Check sheet for the modelled part. Datum: model origin and axes. Units: mm. Face numbers are marked on the shaded views. A direction names the side the tool comes from. Round coordinates to 2 decimals unless told otherwise and drop trailing zeros. Loops run counter-clockwise (first coordinate to the right, second up) from the corner with the lowest first, then second, coordinate; pieces in that order, holes last. Notation, with made-up numbers: (-22, 12) - (-8, 12) arc R26 cw to (-8, 32) - close; hole circle Ø11 at (6, -30.75). An arc over 180 degrees is marked (long way). Answer in a Markdown table with one row per item. Add a question column.
(1) Cross-section at A-A on x = 2. Enter the section's corners in (y, z) (3 decimals), then the cut area to 3 significant figures.
(2) Gauge pin test, flat ends, axial feed: pin 1 (8.5 mm diameter, centred on x = 24, z = 22, fed in from -Y) (3 decimals); pin 2 (5 mm diameter, centred on x = -120, y = -122.125, fed in from -Z); pin 3 (6 mm diameter, centred on x = 24, z = 110, fed in from +Y) (3 decimals); pin 4 (4 mm diameter, centred on x = -24, z = 22, fed in from -Y) (3 decimals). Record the tip position at first contact, or that the pin passes through.
(3) Cross-section at B-B on x = -120. Enter the section's corners in (y, z) (3 decimals).
(4) Cross-section at D-D on z = 41.5. Enter the section's corners in (x, y) (3 decimals).
(5) Access from +Z, -Z, +X, -X, +Y, -Y to the whole of each face (thin tool, end or side, straight path). Record for the marked faces 4, 5, 6, 7 and 8.
(6) Cross-section at C-C on y = 74. Enter the section's corners in (x, z).
(7) Mould release check, pull along X, two halves, no side actions. Record for the marked faces 1, 2 and 3: +X half, -X half, draft (parallel to the pull), parting line (faces both ways), or undercut.
(8) Thickness scan on line 1 along Y through (x, z) = (120, 123) (3 decimals); line 2 along X through (y, z) = (-95, 89.5); line 3 along Z through (x, y) = (-98, 122). Record the ranges inside material, lowest first.
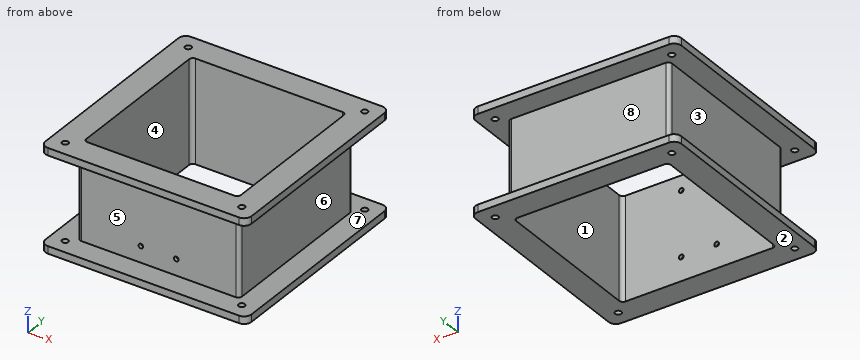
from build123d import *

# Parameters (mm, degrees)
SKETCH_4_W                  = 220
SKETCH_4_H                  = 224.25
SKETCH_4_W_2                = 210
SKETCH_4_H_2                = 214.25
EXTRUDE_7_DEPTH             = 120
SKETCH_7_W                  = 280
SKETCH_7_H                  = 284.25
SKETCH_7_W_2                = 210
SKETCH_7_H_2                = 214.25
EXTRUDE_8_DEPTH             = 10
SKETCH_8_W                  = 280
SKETCH_8_H                  = 284.25
SKETCH_8_W_2                = 210
SKETCH_8_H_2                = 214.25
EXTRUDE_9_DEPTH             = 10
FILLET_5_R                  = 5
FILLET_6_R                  = 10
HOLE_WIZARD_8_4_8_4_1_D     = 8.4
HOLE_WIZARD_6_4_6_4_1_D     = 6.4
HOLE_WIZARD_6_4_6_4_1_DEPTH = 5


with BuildPart() as part:
    # 草图4 → 凸台-拉伸7 (new body)
    with BuildSketch(Plane.XY):
        Rectangle(SKETCH_4_W, SKETCH_4_H)
        Rectangle(SKETCH_4_W_2, SKETCH_4_H_2, mode=Mode.SUBTRACT)
    extrude(amount=EXTRUDE_7_DEPTH)

    # 草图7 → 凸台-拉伸8 (add)
    with BuildSketch(Plane(origin=(0, 0, 0), x_dir=(-1, 0, 0), z_dir=(0, 0, -1))):
        Rectangle(SKETCH_7_W, SKETCH_7_H)
        Rectangle(SKETCH_7_W_2, SKETCH_7_H_2, mode=Mode.SUBTRACT)
    extrude(amount=EXTRUDE_8_DEPTH)

    # 草图8 → 凸台-拉伸9 (add)
    with BuildSketch(Plane.XY.offset(120)):
        Rectangle(SKETCH_8_W, SKETCH_8_H)
        Rectangle(SKETCH_8_W_2, SKETCH_8_H_2, mode=Mode.SUBTRACT)
    extrude(amount=EXTRUDE_9_DEPTH)

    # 圆角5
    fillet_5_edges = [part.edges().sort_by_distance(p)[0] for p in [
        (105, -107.125, 60),
        (105, 107.125, 60),
        (-105, 107.125, 60),
        (-105, -107.125, 60),
        (110, -112.125, 60),
        (-110, -112.125, 60),
        (-110, 112.125, 60),
        (110, 112.125, 60),
    ]]
    fillet(fillet_5_edges, radius=FILLET_5_R)

    # 圆角6
    fillet_6_edges = [part.edges().sort_by_distance(p)[0] for p in [
        (140, 142.125, -5),
        (140, -142.125, -5),
        (-140, -142.125, -5),
        (-140, 142.125, -5),
        (-140, 142.125, 125),
        (-140, -142.125, 125),
        (140, -142.125, 125),
        (140, 142.125, 125),
    ]]
    fillet(fillet_6_edges, radius=FILLET_6_R)

    # Ø8.4 (8.4) 直径孔1 (through all)
    with Locations(Plane(origin=(0, 0, -10), x_dir=(-1, 0, 0), z_dir=(0, 0, -1))):
        with Locations((120, -122.125), (120, 122.125), (-120, 122.125), (-120, -122.125)):
            Hole(HOLE_WIZARD_8_4_8_4_1_D / 2)

    # Ø6.4 (6.4) 直径孔1
    with Locations(Plane(origin=(0, -112.125, 0), x_dir=(-1, 0, 0), z_dir=(0, -1, 0))):
        with Locations((24, -110), (-24, -110), (-24, -22), (24, -22)):
            Hole(HOLE_WIZARD_6_4_6_4_1_D / 2, depth=HOLE_WIZARD_6_4_6_4_1_DEPTH)


solid = part.part
Answers:
| question | item | result |
|---|---|---|
| 1 | outline | (-142.125, -10) - (-107.125, -10) - (-107.125, 130) - (-142.125, 130) - (-142.125, 120) - (-112.125, 120) - (-112.125, 0) - (-142.125, 0) - close; (107.125, -10) - (142.125, -10) - (142.125, 0) - (112.125, 0) - (112.125, 120) - (142.125, 120) - (142.125, 130) - (107.125, 130) - close |
| 1 | area | 2,600 mm^2 |
| 2 | pin 1 | stops at y = -112.125 |
| 2 | pin 2 | passes through |
| 2 | pin 3 | stops at y = 112.125 |
| 2 | pin 4 | stops at y = 107.125 |
| 3 | outline | (-142.125, -10) - (-126.325, -10) - (-126.325, 0) - (-142.125, 0) - close; (-142.125, 120) - (-126.325, 120) - (-126.325, 130) - (-142.125, 130) - close; (-117.925, -10) - (117.925, -10) - (117.925, 0) - (-117.925, 0) - close; (-117.925, 120) - (117.925, 120) - (117.925, 130) - (-117.925, 130) - close; (126.325, -10) - (142.125, -10) - (142.125, 0) - (126.325, 0) - close; (126.325, 120) - (142.125, 120) - (142.125, 130) - (126.325, 130) - close |
| 4 | outline | (-110, -107.125) arc R5 ccw to (-105, -112.125) - (105, -112.125) arc R5 ccw to (110, -107.125) - (110, 107.125) arc R5 ccw to (105, 112.125) - (-105, 112.125) arc R5 ccw to (-110, 107.125) - close; hole (-105, -102.125) arc R5 ccw to (-100, -107.125) - (100, -107.125) arc R5 ccw to (105, -102.125) - (105, 102.125) arc R5 ccw to (100, 107.125) - (-100, 107.125) arc R5 ccw to (-105, 102.125) - close |
| 5 | face 4 | +Z, -Z |
| 5 | face 5 | +X, -X, -Y |
| 5 | face 6 | +X, +Y, -Y |
| 5 | face 7 | none |
| 5 | face 8 | +X, -X, +Y |
| 6 | outline | (-140, -10) - (-105, -10) - (-105, 130) - (-140, 130) - (-140, 120) - (-110, 120) - (-110, 0) - (-140, 0) - close; (105, -10) - (140, -10) - (140, 0) - (110, 0) - (110, 120) - (140, 120) - (140, 130) - (105, 130) - close |
| 7 | face 1 | undercut |
| 7 | face 2 | draft |
| 7 | face 3 | -X half |
| 8 | line 1 | y = -142.125 to -126.325, -117.925 to 117.925, 126.325 to 142.125 |
| 8 | line 2 | x = -110 to -105, 105 to 110 |
| 8 | line 3 | z = -10 to 0, 120 to 130 |
